Check sheet for the drawn part. Datum: minimum x, y, z corner. Units: mm. Give positions to 0.01 mm unless a question says otherwise; leave off trailing zeros. Order: outer loops, then holes, each group sorted by start corner. A loop starts at its lowest first (then second) coordinate and runs counter-clockwise, first axis right, second up. Notation, with made-up numbers: M -6.75,16.25 L 30.25,16.25 A17 ccw 30.25,20.25 Z; hole C -31.5,11.5 d9. An arc over 180 degrees is marked long. Answer in a Markdown table with one row per item. Add a question column.
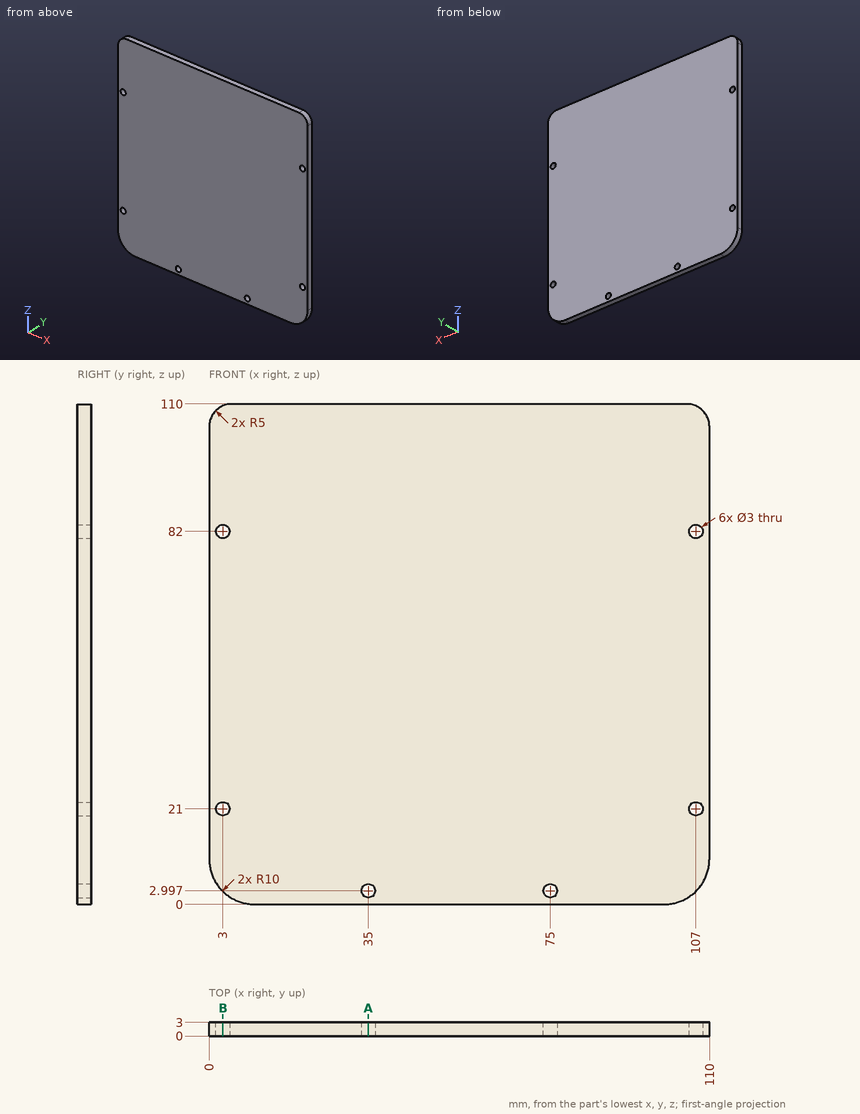
Q1. Cross-section at B-B (x = 3). Record the boundary of the cut face in (y, z), and give its area (3 significant figures).
Q2. Thickness scan on probe 1 along X at (y, z) = (2.2, 82); probe 2 along Z at (x, y) = (35, 1.95); probe 3 along Z at (x, y) = (3, 1.9). Record the ranges inside material, lowest first.
Q3. Cross-section at A-A (x = 35). Record the boundary of the cut face in (y, z).
Values follow:
| question | item | result |
|---|---|---|
| 1 | outline | M 0,2.86 L 3,2.86 L 3,19.5 L 0,19.5 Z; M 0,22.5 L 3,22.5 L 3,80.5 L 0,80.5 Z; M 0,83.5 L 3,83.5 L 3,109.58 L 0,109.58 Z |
| 1 | area | 302 mm² |
| 2 | probe 1 | 0 to 1.5, 4.5 to 105.5, 108.5 to 110 |
| 2 | probe 2 | 0 to 1.5, 4.5 to 110 |
| 2 | probe 3 | 2.86 to 19.5, 22.5 to 80.5, 83.5 to 109.58 |
| 3 | outline | M 0,0 L 3,0 L 3,1.5 L 0,1.5 Z; M 0,4.5 L 3,4.5 L 3,110 L 0,110 Z |
